```python
from build123d import *

# Parameters (mm, degrees)
AUFSATZ_LINEAR_AUSTRAGEN1_DEPTH      = 50
AUFSATZ_LINEAR_AUSTRAGEN1_DEPTH_BACK = 50
SKIZZE4_R                            = 40
SCHNITT_LINEAR_AUSTRAGEN1_DEPTH      = 100
SKIZZE5_W                            = 150
SKIZZE5_H                            = 100
AUFSATZ_LINEAR_AUSTRAGEN2_DEPTH      = 250
VERRUNDUNG2_R                        = 75
SCHNITT_LINEAR_AUSTRAGEN3_REACH      = 492.51
SKIZZE8_W                            = 120
SKIZZE8_H                            = 35
SKIZZE9_R                            = 25
SCHNITT_LINEAR_AUSTRAGEN4_DEPTH      = 20
SKIZZE10_W                           = 150
SKIZZE10_H                           = 130
SCHNITT_LINEAR_AUSTRAGEN5_DEPTH      = 35
VERRUNDUNG3_R                        = 10


with BuildPart() as part:
    # Skizze3 → Aufsatz-Linear austragen1 (new, two sides: drawn at the far end of the back side and taken through both)
    with BuildSketch(Plane(origin=(0, 0, 0), x_dir=(1, 0, 0), z_dir=(0, 1, 0)).offset(-AUFSATZ_LINEAR_AUSTRAGEN1_DEPTH_BACK)):
        Polygon((-265, -40), (-265, 40), (-225, 40), (-225, 100), (225, 100), (225, 40), (265, 40), (265, -40), (225, -40), (225, -100), (-225, -100), (-225, -40), align=None)
    extrude(amount=AUFSATZ_LINEAR_AUSTRAGEN1_DEPTH + AUFSATZ_LINEAR_AUSTRAGEN1_DEPTH_BACK)

    # Skizze4 → Schnitt-Linear austragen1 (cut)
    with BuildSketch(Plane(origin=(0, 50, 0), x_dir=(1, 0, 0), z_dir=(0, 1, 0))):
        with Locations(Location((0, 0, 0), (0, 0, 270))):
            Circle(SKIZZE4_R)
    extrude(amount=-SCHNITT_LINEAR_AUSTRAGEN1_DEPTH, mode=Mode.SUBTRACT)

    # Skizze5 → Aufsatz-Linear austragen2 (add)
    with BuildSketch(Plane.XY.offset(100)):
        Rectangle(SKIZZE5_W, SKIZZE5_H)
    extrude(amount=AUFSATZ_LINEAR_AUSTRAGEN2_DEPTH)

    # Verrundung2
    verrundung2_edges = [part.edges().sort_by_distance(p)[0] for p in [
        (-75, 0, 350),
        (75, 0, 350),
    ]]
    fillet(verrundung2_edges, radius=VERRUNDUNG2_R - 0.0001)  # a hair under: the kernel refuses the full size

    # Schnitt-Linear austragen3: up to this face of the body (flat: up to its plane)
    schnitt_linear_austragen3_end = Plane(part.part.faces().sort_by_distance((-75, 0, 187.50005))[0])
    # Skizze8 → Schnitt-Linear austragen3 (cut, up to the picked face)
    with BuildSketch(Plane(origin=(75, 0, 0), x_dir=(0, 0, -1), z_dir=(1, 0, 0)), mode=Mode.PRIVATE) as schnitt_linear_austragen3_sk1:
        with Locations((-290, 32.5)):
            Rectangle(SKIZZE8_W, SKIZZE8_H)
    schnitt_linear_austragen3_tool1 = split(extrude(schnitt_linear_austragen3_sk1.sketch, amount=-SCHNITT_LINEAR_AUSTRAGEN3_REACH, mode=Mode.PRIVATE), bisect_by=schnitt_linear_austragen3_end, keep=Keep.BOTH, mode=Mode.PRIVATE)
    add(schnitt_linear_austragen3_tool1.solids().sort_by(Axis((75, 32.5, 290), (-1, 0, 0)))[0], mode=Mode.SUBTRACT)

    # Skizze9 → Schnitt-Linear austragen4 (cut)
    with BuildSketch(Plane(origin=(0, 15, 0), x_dir=(1, 0, 0), z_dir=(0, 1, 0))):
        with Locations(Location((0, -275, 0), (0, 0, 180))):
            Circle(SKIZZE9_R)
    extrude(amount=-SCHNITT_LINEAR_AUSTRAGEN4_DEPTH, mode=Mode.SUBTRACT)

    # Skizze10 → Schnitt-Linear austragen5 (cut)
    with BuildSketch(Plane(origin=(0, 50, 0), x_dir=(1, 0, 0), z_dir=(0, 1, 0))):
        with Locations((0, -165)):
            Rectangle(SKIZZE10_W, SKIZZE10_H)
    extrude(amount=-SCHNITT_LINEAR_AUSTRAGEN5_DEPTH, mode=Mode.SUBTRACT)

    # Verrundung3
    verrundung3_edges = [part.edges().sort_by_distance(p)[0] for p in [
        (-75, -17.5, 100),
        (0, 15, 100),
        (-150, -50, 100),
        (225, 0, 100),
        (-225, 0, 100),
        (0, 50, 100),
        (150, -50, 100),
        (75, -17.5, 100),
        (75, -50, 187.50005),
        (-75, -50, 187.50005),
        (53.033037878, -50, 328.033037878),
        (-53.033037878, -50, 328.033037878),
    ]]
    fillet(verrundung3_edges, radius=VERRUNDUNG3_R)


solid = part.part
```
Design review of the part built by this model. Coordinates are the model's own, in mm. A direction names the side the tool comes from. Coordinates: 2 decimals unless noted, no trailing zeros. Loops run counter-clockwise (first coordinate to the right, second up) from the corner with the lowest first, then second, coordinate; pieces in that order, holes last. Notation, with made-up numbers: (-23, 41.5) -> (-6, 41.5) arc R22 cw to (-6, 66.5) -> close; hole circle Ø7 at (7.25, -8.5). An arc over 180 degrees is marked (long way). Answer as a JSON object with one key per item and string values.
Q1. Take a section at A-A on z = 0. Give the boundary of the cut face in (x, y).
Answer block:
{"outline": "(-265, -50) -> (-40, -50) -> (-40, 50) -> (-265, 50) -> close; (40, -50) -> (265, -50) -> (265, 50) -> (40, 50) -> close"}
Q2. The part is to be moulded in two halves that separate along X. For faces 1 (the flat face through (265, -1, -1)), 2 (the flat face through (-245, -1, -40)), 3 (the flat face through (-265, -1, 1)), 4 (the cylindrical face through (-39.05, 0.7, -8.67)), say which applies: +X half, -X half, draft (parallel to the pull), parting line (faces both ways), or undercut.
Answer block:
{"face 1": "+X half", "face 2": "draft", "face 3": "-X half", "face 4": "undercut"}
Q3. Clearance check with flat-ended pins moving along their axes: pin 1 Ø5 at (x, z) = (-156.5, 98) entering from -Y; pin 2 Ø20 at (x, y) = (-250.5, -20.5) entering from -Z; pin 3 Ø4 at (x, z) = (-15, 35) entering from -Y; pin 4 Ø20 at (x, y) = (247.5, -22.5) entering from +Z. State where each tip first meets the part, or that it passes through.
Answer block:
{"pin 1": "stops at y = -48.35", "pin 2": "stops at z = -40", "pin 3": "stops at y = -50", "pin 4": "stops at z = 40"}
Q4. Tool access review of faces 5 (the flat face through (-1, 15, 228)), 6 (the flat face through (-75, -13, 191)), 7 (the flat face through (225, -1, -70)), 8 (the flat face through (75, -13, 191)): name each direction out of +Z, -Z, +X, -X, +Y, -Y from which nothing blocks a thin tool from reaching the whole face with its end or side.
Answer block:
{"face 5": "+Z, +X, -X, +Y", "face 6": "+Z, -X, +Y, -Y", "face 7": "-Z, +X, +Y, -Y", "face 8": "+Z, +X, +Y, -Y"}
Q5. To check wall thickness, follow L1, parallel to X at y = 2, z = 0; L2, parallel to Z at x = 132.5, y = -28; L3, parallel to Z at x = 12, y = -9.5. State the ranges of each line that lie inside material, in increasing order.
Answer block:
{"L1": "x = -265 to -40, 40 to 265", "L2": "z = -100 to 100", "L3": "z = -100 to -38.16, 38.16 to 349.03"}
Q6. Take a section at C-C on z = 178. Give the boundary of the cut face in (x, y), plus the area to 3 significant figures.
Answer block:
{"outline": "(-75, -40) arc R10 ccw to (-65, -50) -> (65, -50) arc R10 ccw to (75, -40) -> (75, 15) -> (-75, 15) -> close", "area": "9,710 mm^2"}
Q7. Take a section at D-D on x = 134. Give the boundary of the cut face in (y, z), plus the area to 3 significant figures.
Answer block:
{"outline": "(-50, -100) -> (50, -100) -> (50, 90) arc R10 ccw to (40, 100) -> (-40, 100) arc R10 ccw to (-50, 90) -> close", "area": "20,000 mm^2"}
